Work out the finished part from the listing and answer in its coordinate system (mm). A direction names the side the tool comes from. Round coordinates to 2 decimals unless told otherwise and drop trailing zeros. Order: outer loops, then holes, each group sorted by start corner. A loop starts at its lowest first (then second) coordinate and runs counter-clockwise, first axis right, second up. Notation, with made-up numbers: M -20,-9 L 9,-9 A14 cw 9,-2 Z; hole C 58.25,30 d2. An arc over 180 degrees is marked long. Return JSON: item names as keys, results as strings.
from build123d import *

# Parameters (mm, degrees)
SKETCH1_W           = 50.8
SKETCH1_H           = 76.2
SKETCH1_W_2         = 38.1
SKETCH1_H_2         = 63.5
BOSS_EXTRUDE1_DEPTH = 279.4
SKETCH2_R           = 6.35
CUT_EXTRUDE1_DEPTH  = 77.2
SKETCH3_W           = 50.8
SKETCH3_H           = 38.1
BOSS_EXTRUDE2_DEPTH = 2.54


with BuildPart() as part:
    # Sketch1 → Boss-Extrude1 (new body, symmetric)
    with BuildSketch(Plane(origin=(0, 0, 0), x_dir=(1, 0, 0), z_dir=(0, 1, 0))):
        Rectangle(SKETCH1_W, SKETCH1_H)
        Rectangle(SKETCH1_W_2, SKETCH1_H_2, mode=Mode.SUBTRACT)
    extrude(amount=BOSS_EXTRUDE1_DEPTH, both=True)

    # Sketch2 → Cut-Extrude1 (cut, through all)
    with BuildSketch(Plane.XY.offset(38.1)):
        Circle(SKETCH2_R)
    extrude(amount=-CUT_EXTRUDE1_DEPTH, mode=Mode.SUBTRACT)

    # Sketch3 → Boss-Extrude2 (add)
    with BuildSketch(Plane(origin=(0, 0, -38.1), x_dir=(-1, 0, 0), z_dir=(0, 0, -1))):
        with Locations((0, -208.386065816)):
            Rectangle(SKETCH3_W, SKETCH3_H)
    boss_extrude2 = extrude(amount=BOSS_EXTRUDE2_DEPTH)

    # Mirror1: Boss-Extrude2 across plane
    add(boss_extrude2.mirror(Plane.ZX))


solid = part.part
Item 1: Find section B-B (z = -13). Determine the outline of the cut face in (x, y), plus the area to 3 significant figures.
Output:
{"outline": "M -25.4,-279.4 L -19.05,-279.4 L -19.05,279.4 L -25.4,279.4 Z; M 19.05,-279.4 L 25.4,-279.4 L 25.4,279.4 L 19.05,279.4 Z", "area": "7,100 mm^2"}
Item 2: Find section A-A (x = 0). Determine the outline of the cut face in (y, z).
Output:
{"outline": "M -279.4,-38.1 L -227.44,-38.1 L -227.44,-40.64 L -189.34,-40.64 L -189.34,-38.1 L -6.35,-38.1 L -6.35,-31.75 L -279.4,-31.75 Z; M -279.4,31.75 L -6.35,31.75 L -6.35,38.1 L -279.4,38.1 Z; M 6.35,-38.1 L 189.34,-38.1 L 189.34,-40.64 L 227.44,-40.64 L 227.44,-38.1 L 279.4,-38.1 L 279.4,-31.75 L 6.35,-31.75 Z; M 6.35,31.75 L 279.4,31.75 L 279.4,38.1 L 6.35,38.1 Z"}
Item 3: Which of the six approach directions +Z, -Z, +X, -X, +Y, -Y give full straight-line access (tool end or side, diameter ignored) to faces 1 (the flat face through (8, 4, 31.75)), 2 (the flat face through (-6, 3, -38.1)), 3 (the flat face through (0, -253, -38.1))?
Output:
{"face 1": "+Y, -Y", "face 2": "-Z, +X, -X", "face 3": "-Z, +X, -X, -Y"}
Item 4: Each of these flat-tipped pins is pushed along its axis until it touches: pin 1 (1.3 mm diameter, centred on x = -7, z = -39, fed in from +Y); pin 2 (1.5 mm diameter, centred on x = -17, y = -54.5, fed in from -Z); pin 3 (1.3 mm diameter, centred on x = 2.5, z = -40, fed in from -Y). Where does it stop, or does it pass through?
Output:
{"pin 1": "stops at y = 227.44", "pin 2": "stops at z = -38.1", "pin 3": "stops at y = -227.44"}
Item 5: Consider line 1 along X through (y, z) = (242.5, 31.5); line 2 along Y through (x, z) = (0, 34.75); line 3 along Z through (x, y) = (-3.5, -123). Determine where each line is inside the solid, lowest interval first. Write a range as [from, to].
Output:
{"line 1": "x = [-25.4, -19.05], [19.05, 25.4]", "line 2": "y = [-279.4, -6.35], [6.35, 279.4]", "line 3": "z = [-38.1, -31.75], [31.75, 38.1]"}
Item 6: Find section D-D (y = 0). Determine the outline of the cut face in (x, z), plus the area to 3 significant figures.
Output:
{"outline": "M -25.4,-38.1 L -6.35,-38.1 L -6.35,-31.75 L -19.05,-31.75 L -19.05,31.75 L -6.35,31.75 L -6.35,38.1 L -25.4,38.1 Z; M 6.35,-38.1 L 25.4,-38.1 L 25.4,38.1 L 6.35,38.1 L 6.35,31.75 L 19.05,31.75 L 19.05,-31.75 L 6.35,-31.75 Z", "area": "1,290 mm^2"}
Item 7: Find section C-C (y = -164). Determine the outline of the cut face in (x, z).
Output:
{"outline": "M -25.4,-38.1 L 25.4,-38.1 L 25.4,38.1 L -25.4,38.1 Z; hole M -19.05,-31.75 L 19.05,-31.75 L 19.05,31.75 L -19.05,31.75 Z"}
Item 8: The mould has two halves that part along Y. Classify faces 4 (the cylindrical face through (-1.38, -6.2, -34.88)), 5 (the flat face through (5.3, 3.9, 38.1)), 6 (the cylindrical face through (-1.38, -6.2, 34.97)), 7 (the flat face through (22, 279.4, -1)): pulls with the +Y half, pulls with the -Y half, needs draft (parallel to the pull), parting line crosses it, or undercut.
Output:
{"face 4": "undercut", "face 5": "needs draft", "face 6": "undercut", "face 7": "pulls with the +Y half"}
